For this review, take the finished solid that the model builds, in its own axes (mm). Face numbers are marked on the shaded views. A direction names the side the tool comes from. Give positions to 0.01 mm unless a question says otherwise; leave off trailing zeros. Order: outer loops, then holes, each group sorted by start corner. A loop starts at its lowest first (then second) coordinate and runs counter-clockwise, first axis right, second up. Notation, with made-up numbers: (77.5, -31) -> (81.5, -31) arc R17 cw to (81.5, -20) -> close; hole circle Ø3 at (68.5, 62.5). An arc over 180 degrees is marked (long way). Return JSON: item names as keys, results as strings. Group by question number.
1) Add section D-D (y = 137). Give the boundary of the cut face in (x, z).
2) The part is to be moulded in two halves that separate along Y. For the marked faces 3 and 4, say which applies: released by +Y, released by -Y, zero draft, split by the parting line, or undercut.
3) Add section B-B (z = 135). Give the boundary of the cut face in (x, y), then the cut area to 3 significant figures.
4) Add section C-C (x = 12.5). Give the boundary of the cut face in (y, z), then the cut area to 3 significant figures.
5) To check wall thickness, follow line 1 along Y through (x, z) = (22, 244); line 2 along Y through (x, z) = (37.25, 261); line 3 along X through (y, z) = (146, 107). State the ranges of each line that lie inside material, in increasing order.
6) For the marked faces 1 and 2, list the 3-axis set-ups (+Z, -Z, +X, -X, +Y, -Y) from which the entire face can be reached by the end or side of a thin tool; tool diameter is ignored.
7) Insertion check: P1, Ø8, axis at x = 14, y = 77, coming from the -Z side; P2, Ø5, axis at x = 14.5, y = 66, coming from the -Z side; P3, Ø8, axis at y = 113.5, z = 200, coming from the -X side. Each pin has a flat end and moves straight along its axis. Give the tip position at first contact, or say it passes through.
8) Add section A-A (y = 80). Give the boundary of the cut face in (x, z), then the cut area to 3 significant figures.
Autodesk Inventor part; units mm, degrees
ref_plane "YZ Plane" through (0, 0, 0) normal (1, 0, 0) x (0, 1, 0)
ref_plane "XZ Plane" through (0, 0, 0) normal (0, 1, 0) x (-1, 0, 0)
ref_plane "XY Plane" through (0, 0, 0) normal (0, 0, 1) x (1, 0, 0)
sketch "Sketch1" plane through (0, 0, 0) normal (0, 1, 0) x (-1, 0, 0)
  line L0 (0, 279.3478) -> (-39.1304, 279.3478)
  line L1 (-39.1304, 279.3478) -> (-39.1304, -270.6522)
  line L2 (-39.1304, -270.6522) -> (0, -270.6522)
  line L3 (0, -270.6522) -> (0, 279.3478)
  line L4 (-39.1304, 279.3478) -> (-29.1304, 279.3478)
  line L5 (-29.1304, 254.3478) -> (-39.1304, 254.3478)
  line L6 (-39.1304, 254.3478) -> (-39.1304, 279.3478)
  line L7 (-39.1304, -270.6522) -> (-29.1304, -270.6522)
  line L8 (-29.1304, -245.6522) -> (-39.1304, -245.6522)
  line L9 (-39.1304, -245.6522) -> (-39.1304, -270.6522)
  point P0 (0, 0)
  point P1 (-39.1304, 254.3478)
  point P2 (-39.1304, -245.6522)
  dimension "d0" = 550
  dimension "d4" = 25
  dimension "d5" = 25
  dimension "d28" = 39.1304
extrude "Extrusion1" add sketch "Sketch1" along normal blind 160
sketch "Sketch2" plane through (0, 0, 279.3478) normal (0, 0, 1) x (1, 0, 0)
  line L0 (0, 160) -> (39.1304, 160)
  line L1 (0, 160) -> (39.1304, 160)
  line L2 (39.1304, 160) -> (39.1304, 0)
  line L3 (39.1304, 0) -> (0, 0)
  line L4 (0, 0) -> (0, 160)
  line L5 (39.1304, 160) -> (39.1304, 160)
  line L6 (39.1304, 160) -> (39.1304, 115)
  line L7 (39.1304, 115) -> (39.1304, 115)
  line L8 (39.1304, 115) -> (39.1304, 160)
  line L9 (39.1304, 0) -> (39.1304, 0)
  line L10 (39.1304, 0) -> (39.1304, 45)
  line L11 (39.1304, 45) -> (39.1304, 45)
  line L12 (39.1304, 45) -> (39.1304, 0)
  circle A0 centre (39.1304, 80) radius 18
  line L13 (31.1304, 75) -> (39.1304, 75)
  line L14 (39.1304, 75) -> (39.1304, 98)
  line L15 (39.1304, 98) -> (31.1304, 98)
  line L16 (31.1304, 98) -> (31.1304, 75)
  line L17 (31.1304, 75) -> (39.1304, 75)
  line L18 (39.1304, 75) -> (39.1304, 62)
  line L19 (39.1304, 62) -> (31.1304, 62)
  line L20 (31.1304, 62) -> (31.1304, 75)
  line L21 (39.1304, 0) -> (39.1304, 160)
  line L22 (0, 160) -> (9.1304, 160)
  line L23 (9.1304, 160) -> (9.1304, 0)
  line L24 (9.1304, 0) -> (0, 0)
  line L25 (0, 0) -> (0, 160)
  line L26 (19.1304, 98) -> (-11, 98)
  line L27 (-11, 98) -> (-11, 62)
  line L28 (-11, 62) -> (19.1304, 62)
  line L29 (19.1304, 62) -> (19.1304, 98)
  line L30 (-8, 54) -> (24, 54)
  line L31 (24, 54) -> (24, 0)
  line L32 (24, 0) -> (-8, 0)
  line L33 (-8, 0) -> (-8, 54)
  line L34 (-8, 160) -> (24, 160)
  line L35 (24, 160) -> (24, 106)
  line L36 (24, 106) -> (-8, 106)
  line L37 (-8, 106) -> (-8, 160)
  point P0 (0, 0)
  point P1 (39.1304, 115)
  point P2 (39.1304, 160)
  point P3 (39.1304, 45)
  point P4 (39.1304, 0)
  point P5 (39.1304, 115)
  point P6 (0, 98)
  point P7 (0, 62)
  point P8 (9.1304, 98)
  point P9 (9.1304, 106)
  point P10 (9.1304, 54)
  point P11 (9.1304, 62)
  dimension "d6" = 0
  dimension "d7" = 45
  dimension "d8" = 45
  dimension "d9" = 8
  dimension "d10" = 36
  dimension "d11" = 80
  dimension "d12" = 80
  dimension "d15" = 30
  dimension "d34" = 12
extrude "Extrusion2" cut sketch "Sketch2" against normal up to surface (550 mm away) contours L0 L23 L36 L4 | L0 L35 L36 L23 | L36 L23 L26 L4 | L26 L23 L28 L4 | L26 L29 L28 L23 | L28 L23 L30 L4 | L30 L23 L3 L4 | L2 L13 L16 A0 | A0 L16 L15 | L30 L31 L3 L23 | L2 A0 L20 L13 | L19 L20 A0
sketch "Sketch5" plane through (39.1304, 160, 279.3478) normal (1, 0, 0) x (0, 0, -1)
  line L0 (0, -62) -> (0, 0)
  line L1 (0, -160) -> (550, -160)
  line L2 (0, 0) -> (214, 0)
  line L3 (214, 0) -> (214, -160)
  line L4 (214, -160) -> (0, -160)
  line L5 (0, -160) -> (0, 0)
  circle A0 centre (214, -80) radius 35
  line L6 (214, 0) -> (550, 0)
  line L7 (550, 0) -> (550, -160)
  line L8 (550, -160) -> (214, -160)
  line L9 (214, -160) -> (214, 0)
  point P0 (279.3478, -160)
  point P1 (214, -45)
  point P2 (214, -115)
  dimension "d30" = 160
  dimension "d31" = 70
extrude "Extrusion4" cut sketch "Sketch5" against normal blind 100 contours L6 L7 L1 L3 A0 | A0 L3 | L3 A0
sketch "Sketch6" plane through (19.1304, 62, 279.3478) normal (-1, 0, 0) x (0, 0, 1)
  line L0 (0, 52.95) -> (-60, 52.95)
  line L1 (-60, 52.95) -> (-60, -16.95)
  line L2 (-60, -16.95) -> (0, -16.95)
  line L3 (0, -16.95) -> (0, 52.95)
  line L4 (0, -62) -> (-214, -62)
  line L5 (-214, 98) -> (0, 98)
  point P0 (-279.3478, -62)
  dimension "d43" = 45.05
  dimension "d44" = 45.05
  dimension "d45" = 60
extrude "Extrusion5" add sketch "Sketch6" along normal mid plane 20
sketch "Sketch7" plane through (24, 0, 279.3478) normal (0, 0, 1) x (1, 0, 0)
  point P0 (-24, 0)
sketch "Sketch8" plane through (39.1304, 0, 279.3478) normal (1, 0, 0) x (0, 0, -1)
  line L0 (0, 0) -> (0, 62)
  line L1 (0, 52) -> (50, 52)
  line L2 (50, 52) -> (50, 108)
  line L3 (50, 108) -> (0, 108)
  line L4 (0, 108) -> (0, 52)
  line L5 (183.9833, 62) -> (0, 62)
  line L6 (0, 98) -> (183.9833, 98)
  point P0 (279.3478, 0)
  dimension "d38" = 10
  dimension "d39" = 10
  dimension "d40" = 50
extrude "Extrusion6" cut sketch "Sketch8" against normal blind 20
sketch "Sketch9" plane through (31.1304, 80, 65.3478) normal (1, 0, 0) x (0, 0, -1)
  line L0 (-164, 18) -> (-164, -18)
  line L1 (-154, -18) -> (-30.0167, -18)
  line L2 (-164, 18) -> (-169, 18)
  line L3 (-169, 18) -> (-169, -18)
  line L4 (-169, -18) -> (-164, -18)
  line L5 (-164, -18) -> (-164, 18)
  point P0 (65.3478, -80)
  point P1 (-214, -18)
extrude "Extrusion7" add sketch "Sketch9" against normal blind 10
sketch "Sketch10" plane through (9.1304, 45.05, 279.3478) normal (-1, 0, 0) x (0, 0, 1)
  line L0 (-60, 52.95) -> (-60, 16.95)
  line L1 (-60, 26.95) -> (-65, 26.95)
  line L2 (-65, 26.95) -> (-65, 42.95)
  line L3 (-65, 42.95) -> (-60, 42.95)
  line L4 (-60, 42.95) -> (-60, 26.95)
  line L5 (-60, 16.95) -> (-183.9833, 16.95)
  line L6 (-60, 52.95) -> (-183.9833, 52.95)
  point P0 (-279.3478, -45.05)
  point P1 (-60, 42.95)
  dimension "d48" = 10
  dimension "d49" = 10
extrude "Extrusion8" add sketch "Sketch10" against normal blind 10
properties part number "MainRails" material "Aluminum 6061"
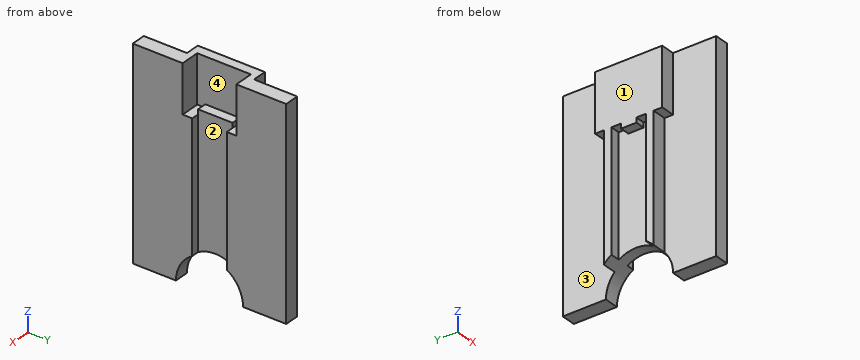
Evaluation:
{
 "1": {"outline": "(24, 65.35) -> (39.13, 65.35) -> (39.13, 279.35) -> (24, 279.35) -> close"},
 "2": {"face 3": "zero draft", "face 4": "undercut"},
 "3": {"outline": "(9.13, 54) -> (24, 54) -> (24, 0) -> (39.13, 0) -> (39.13, 62) -> (31.13, 62) -> (31.13, 98) -> (39.13, 98) -> (39.13, 160) -> (24, 160) -> (24, 106) -> (9.13, 106) -> (9.13, 98) -> (19.13, 98) -> (19.13, 62) -> (9.13, 62) -> close", "area": "2,550 mm^2"},
 "4": {"outline": "(45.05, 219.35) -> (54, 219.35) -> (54, 88.78) arc R35 cw to (62, 95.36) -> (62, 219.35) -> (72, 219.35) -> (72, 214.35) -> (88, 214.35) -> (88, 219.35) -> (98, 219.35) -> (98, 95.36) arc R35 cw to (106, 88.78) -> (106, 219.35) -> (114.95, 219.35) -> (114.95, 279.35) -> (45.05, 279.35) -> close", "area": "6,310 mm^2"},
 "5": {"line 1": "45.05 to 52, 108 to 114.95", "line 2": "0 to 52, 108 to 160", "line 3": "24 to 39.13"},
 "6": {"face 1": "+Z, -Z, -X, +Y, -Y", "face 2": "+Z, -Z, +X"},
 "7": {"P1": "z = 214.35", "P2": "z = 219.35", "P3": "x = 24"},
 "8": {"outline": "(9.13, 214.35) -> (19.13, 214.35) -> (19.13, 100.35) -> (31.13, 100.35) -> (31.13, 234.35) -> (21.13, 234.35) -> (21.13, 229.35) -> (19.13, 229.35) -> (19.13, 279.35) -> (9.13, 279.35) -> close", "area": "2,250 mm^2"}
}
